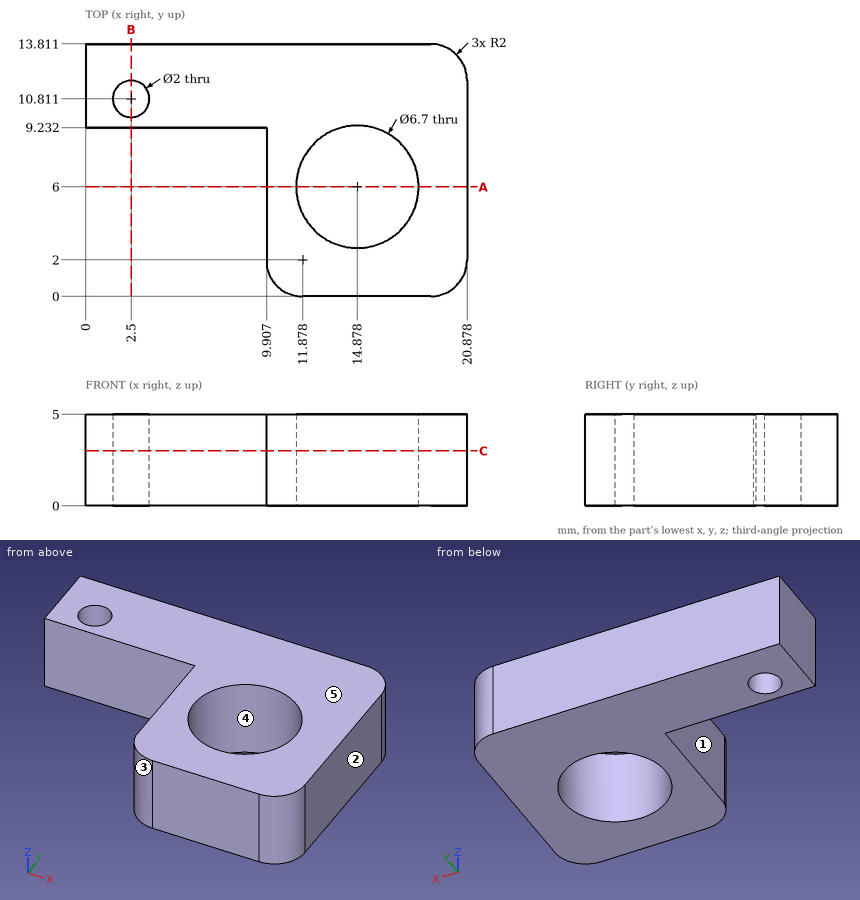
The drawing under review shows one solid part. Ordinate dimensions are in mm from its lowest x, y, z. A direction names the side the tool comes from. Coordinates: 2 decimals unless noted, no trailing zeros. Loops run counter-clockwise (first coordinate to the right, second up) from the corner with the lowest first, then second, coordinate; pieces in that order, holes last. Notation, with made-up numbers: (80, -4) -> (117, -4) arc R34 cw to (117, 34) -> close; hole circle Ø2 at (36.25, 68.25). An arc over 180 degrees is marked (long way). Answer as a JSON object with one key per item and string values.
Q1. The part is to be moulded in two halves that separate along Y. For the marked faces 3, 4 and 5, say which applies: +Y half, -Y half, draft (parallel to the pull), parting line (faces both ways), or undercut.
Answer block:
{"face 3": "-Y half", "face 4": "undercut", "face 5": "draft"}
Q2. Clearance check with flat-ended pins moving along their axes: pin 1 Ø3 at (x, z) = (15, 2) entering from -Y; pin 2 Ø2.5 at (x, z) = (6.5, 2) entering from -Y; pin 3 Ø4 at (x, y) = (14.88, 6) entering from -Z; pin 4 Ø1.5 at (y, z) = (4.5, 2.5) entering from -X. State where each tip first meets the part, or that it passes through.
Answer block:
{"pin 1": "stops at y = 0", "pin 2": "stops at y = 9.23", "pin 3": "passes through", "pin 4": "stops at x = 9.91"}
Q3. To check wall thickness, follow L1, parallel to X at y = 2.25, z = 4.3; L2, parallel to Y at x = 6.75, z = 1.95; L3, parallel to Y at x = 2.5, z = 1.1. State the ranges of each line that lie inside material, in increasing order.
Answer block:
{"L1": "x = 9.91 to 20.88", "L2": "y = 9.23 to 13.81", "L3": "y = 9.23 to 9.81, 11.81 to 13.81"}
Q4. Take a section at B-B on x = 2.5. Give the boundary of the cut face in (y, z).
Answer block:
{"outline": "(9.23, 0) -> (9.81, 0) -> (9.81, 5) -> (9.23, 5) -> close; (11.81, 0) -> (13.81, 0) -> (13.81, 5) -> (11.81, 5) -> close"}
Q5. Take a section at C-C on z = 3. Give the boundary of the cut face in (x, y).
Answer block:
{"outline": "(0, 9.23) -> (9.91, 9.23) -> (9.91, 1.66) arc R2 ccw to (11.88, 0) -> (18.88, 0) arc R2 ccw to (20.88, 2) -> (20.88, 11.81) arc R2 ccw to (18.88, 13.81) -> (0, 13.81) -> close; hole circle Ø2 at (2.5, 10.81); hole circle Ø6.7 at (14.88, 6)"}
Q6. Tool access review of the marked faces 1 and 2: name each direction out of +Z, -Z, +X, -X, +Y, -Y from which nothing blocks a thin tool from reaching the whole face with its end or side.
Answer block:
{"face 1": "+Z, -Z, -X, -Y", "face 2": "+Z, -Z, +X, +Y, -Y"}
Q7. Take a section at A-A on y = 6. Give the boundary of the cut face in (x, z).
Answer block:
{"outline": "(9.91, 0) -> (11.53, 0) -> (11.53, 5) -> (9.91, 5) -> close; (18.23, 0) -> (20.88, 0) -> (20.88, 5) -> (18.23, 5) -> close"}
